from build123d import *

# Parameters (mm, degrees)
MAIN_BODY_DEPTH   = 5
SCREW_HOLES_REACH = 18.771
SCHIZZO2_R        = 1.8


with BuildPart() as part:
    # Schizzo1 → Main body (new, symmetric)
    with BuildSketch(Plane.XY):
        with BuildLine():
            Line((-12.5, -5), (12.5, -5))
            Line((12.5, -5), (12.5, 5))
            Line((12.5, 5), (4.09, 5))
            ThreePointArc((4.09, 5), (0, 0.91), (-4.09, 5))
            Line((-4.09, 5), (-12.5, 5))
            Line((-12.5, 5), (-12.5, -5))
        make_face()
    extrude(amount=MAIN_BODY_DEPTH, both=True)

    # Schizzo2 → screw holes (cut, up to next)
    with BuildSketch(Plane.XZ.offset(5), mode=Mode.PRIVATE) as screw_holes_sk1:
        with Locations(Location((-7, 0, 0), (0, 0, 270))):
            Circle(SCHIZZO2_R)
    screw_holes_tool1 = extrude(screw_holes_sk1.sketch, amount=-SCREW_HOLES_REACH, mode=Mode.PRIVATE) & part.part
    # Schizzo2 → screw holes (cut, up to next)
    with BuildSketch(Plane.XZ.offset(5), mode=Mode.PRIVATE) as screw_holes_sk2:
        with Locations(Location((7, 0, 0), (0, 0, 180))):
            Circle(SCHIZZO2_R)
    screw_holes_tool2 = extrude(screw_holes_sk2.sketch, amount=-SCREW_HOLES_REACH, mode=Mode.PRIVATE) & part.part
    add(screw_holes_tool1.solids().sort_by_distance((-7, -5, 0))[0], mode=Mode.SUBTRACT)
    add(screw_holes_tool2.solids().sort_by_distance((7, -5, 0))[0], mode=Mode.SUBTRACT)


solid = part.part
For this review, take the finished solid that the model builds, in its own axes (mm). Give positions to 0.01 mm unless a question says otherwise; leave off trailing zeros. Loops run counter-clockwise (first coordinate to the right, second up) from the corner with the lowest first, then second, coordinate; pieces in that order, holes last.
Item 1: Draft analysis for pull direction Z (two halves, no side actions). For faces 1 (the flat face through (0, 0, 5)), 2 (the cylindrical face through (0.09, 0.91, 0.07)), 3 (the cylindrical face through (8.8, -0.07, -0.08)), 4 (the flat face through (0, 0, -5)), state which applies: +Z half, -Z half, draft (parallel to the pull), parting line (faces both ways), or undercut.
Item 2: Insertion check: pin 1 (1 mm diameter, centred on x = 2, z = -2.5, fed in from +Y). The pin has a flat end and moves straight along its axis. Give the tip position at first contact, or say it passes through.
Item 3: Take a section at A-A, the plane z = 0. State the section outline as (x, y) points, and give its area (3 significant figures).
Item 4: For line 1 along Z through (x, y) = (7, -0.5); line 2 along X through (y, z) = (2, 4.75); line 3 along Z through (x, y) = (8.25, 4.5), list the stretches that pass through material, from the lowest coordinate up.
Item 5: Take a section at C-C, the plane x = 7. State the section outline as (y, z) points, and give its area (3 significant figures).
Item 6: Take a section at D-D, the plane y = -4.5. State the section outline as (x, z) points, and give its area (3 significant figures).
Item 7: Take a section at B-B, the plane y = 2.75. State the section outline as (x, z) points.
Calculated:
1. face 1: +Z half
1. face 2: draft
1. face 3: undercut
1. face 4: -Z half
2. pin 1: stops at y = 1.76
3. outline: (-12.5, -5) - (-8.8, -5) - (-8.8, 5) - (-12.5, 5) - close; (-5.2, -5) - (5.2, -5) - (5.2, 5) - (4.09, 5) arc R4.09 cw to (-4.09, 5) - (-5.2, 5) - close; (8.8, -5) - (12.5, -5) - (12.5, 5) - (8.8, 5) - close
3. area: 152 mm2
4. line 1: z = -5 to -1.8, 1.8 to 5
4. line 2: x = -12.5 to -2.78, 2.78 to 12.5
4. line 3: z = -5 to -1.3, 1.3 to 5
5. outline: (-5, -5) - (5, -5) - (5, -1.8) - (-5, -1.8) - close; (-5, 1.8) - (5, 1.8) - (5, 5) - (-5, 5) - close
5. area: 64.0 mm2
6. outline: (-12.5, -5) - (12.5, -5) - (12.5, 5) - (-12.5, 5) - close; hole circle Ø3.6 at (-7, 0); hole circle Ø3.6 at (7, 0)
6. area: 230 mm2
7. outline: (-12.5, -5) - (-3.42, -5) - (-3.42, 5) - (-12.5, 5) - close; (3.42, -5) - (12.5, -5) - (12.5, 5) - (3.42, 5) - close; hole circle Ø3.6 at (-7, 0); hole circle Ø3.6 at (7, 0)
